Part print with two shaded views. Sizes in mm from the minimum x, y, z corner. A direction names the side the tool comes from. Coordinates: 2 decimals unless noted, no trailing zeros. Write each loop counter-clockwise with the first axis right and the second up, starting at its lowest first coordinate (ties: lowest second). Pieces come first, ordered by that corner, then holes. Notation, with made-up numbers: (6, 86.25) - (11, 86.25) arc R27 cw to (11, 118.25) - close; hole circle Ø11 at (-9, 10.25). An arc over 180 degrees is marked (long way). One line per question, with ' | ' between items. Start each with the question number.
1. Probe line 1 (Y direction, x = 25, z = 15) (1 decimal); line 2 (Y direction, x = 31.5, z = 15) (1 decimal); line 3 (X direction, y = 63, z = 22.5). List the from-to ranges inside material, lowest first.
2. Band-saw the part on B-B, the plane y = 61.5. Write the cut outline in (x, z) (1 decimal).
3. Flat gauge pins, fed straight in: P1, Ø6, axis at y = 7.5, z = 21, coming from the -X side; P2, Ø7, axis at y = 63.52, z = 15, coming from the +X side; P3, Ø2, axis at y = 15, z = 19, coming from the +X side. Where does each tip first touch, or does it go through?
4. Which spindle directions (+Z, -Z, +X, -X, +Y, -Y) get a long thin tool onto all of the face, cutting with end or side? Do the marked faces 1, 2, 3, 4 and 5. Say none if no direction does.
5. Two-plate mould, pull along Y, no slides. Class the marked faces 6, 7 and 8: +Y half, -Y half, draft (parallel to the pull), parting line (faces both ways), or undercut.
6. Band-saw the part on C-C, the plane z = 25.5. Write the cut outline in (x, y) (1 decimal).
7. Band-saw the part on A-A, the plane x = 23.5. Write the cut outline in (y, z) (1 decimal), then the cut area to 3 significant figures.
8. Band-saw the part on D-D, the plane x = 34.5. Write the cut outline in (y, z) (1 decimal).
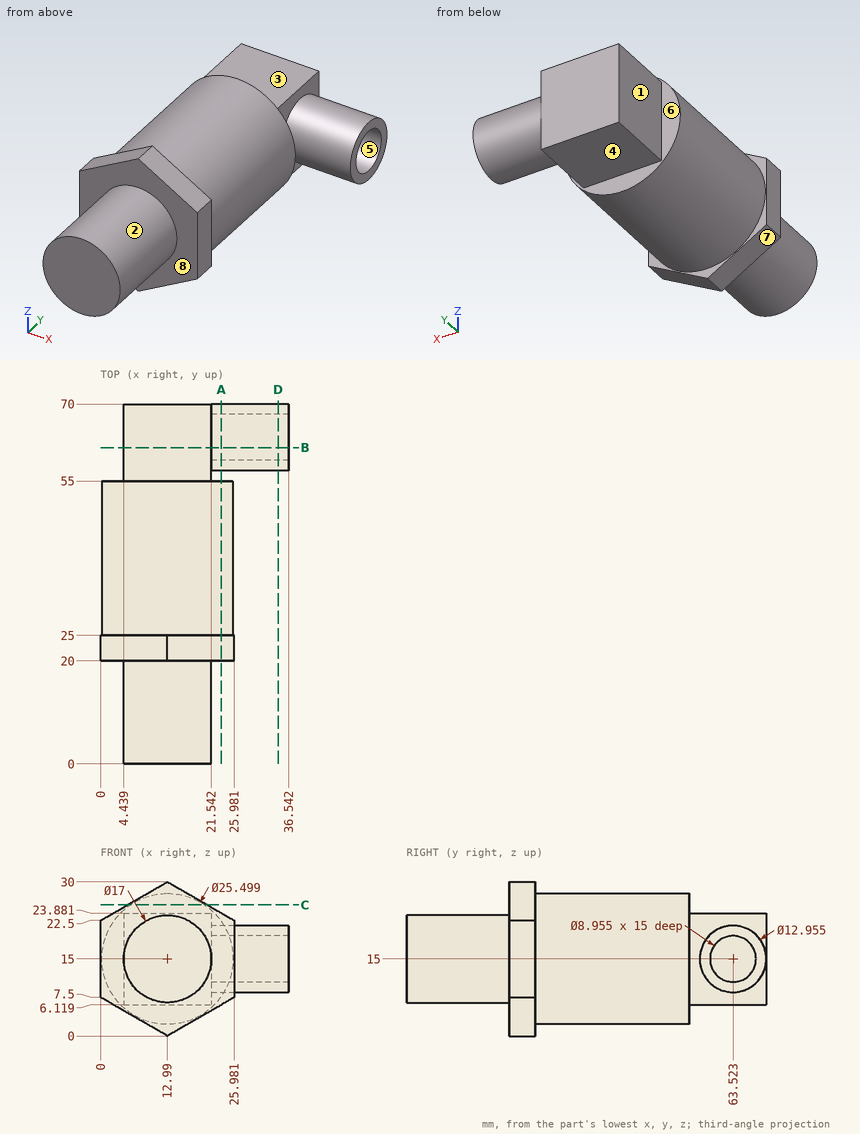
Filled in:
1) line 1: y = 20 to 55, 57 to 59, 68 to 70 | line 2: y = 57 to 59, 68 to 70 | line 3: x = 4.44 to 21.54
2) outline: (4.4, 6.1) - (21.5, 6.1) - (21.5, 8.8) - (36.5, 8.8) - (36.5, 11) - (21.5, 11) - (21.5, 19) - (36.5, 19) - (36.5, 21.2) - (21.5, 21.2) - (21.5, 23.9) - (4.4, 23.9) - close
3) P1: stops at x = 5.04 | P2: stops at x = 21.54 | P3: stops at x = 20.94
4) face 1: +Z, -Z, -X, +Y | face 2: -Y | face 3: +Z, +X, -X, +Y | face 4: -Z, +X, -X, +Y | face 5: +X
5) face 6: undercut | face 7: draft | face 8: -Y half
6) outline: (5.2, 20) - (20.8, 20) - (20.8, 25) - (20.2, 25) - (20.2, 55) - (5.8, 55) - (5.8, 25) - (5.2, 25) - close
7) outline: (20, 6.1) - (25, 6.1) - (25, 7.8) - (55, 7.8) - (55, 22.2) - (25, 22.2) - (25, 23.9) - (20, 23.9) - close; circle Ø13 at (63.5, 15); hole circle Ø9 at (63.5, 15) | area: 591 mm²
8) outline: circle Ø13 at (63.5, 15); hole circle Ø9 at (63.5, 15)
